Can you work these out from the model? Positions are in its coordinate system, mm. A direction names the side the tool comes from. Give positions to 0.01 mm unless a question says otherwise; leave off trailing zeros. Write each loop counter-clockwise with the first axis right and the second up, starting at its lowest first coordinate (ties: lowest second). Pieces come first, ordered by that corner, then holes.
Autodesk Inventor part; units mm, degrees
ref_plane "YZ Plane" through (0, 0, 0) normal (1, 0, 0) x (0, 1, 0)
ref_plane "XZ Plane" through (0, 0, 0) normal (0, 1, 0) x (-1, 0, 0)
ref_plane "XY Plane" through (0, 0, 0) normal (0, 0, 1) x (1, 0, 0)
sketch "Sketch1" plane through (0, 0, 0) normal (0, 1, 0) x (-1, 0, 0)
  circle A0 centre (0, 0) radius 4.25
  dimension "d0" = 8.5
extrude "Extrusion1" add sketch "Sketch1" along normal blind 2.5
sketch "Sketch2" plane through (0, 0, 0) normal (0, -1, 0) x (1, 0, 0)
  circle A0 centre (0, 0) radius 5.5
  dimension "d3" = 11
extrude "Extrusion2" add sketch "Sketch2" along normal blind 2.7
fillet "Fillet1" radius 1 1 edges at (4.25, 2.5, 0)
chamfer "Chamfer1" distance 2 angle 45 1 edges at (-5.5, -2.7, 0)
properties part number "button_round_3DPrint"
1) Suppose I cut it at B-B on z = 0. Write out the boundary of the cut face in (x, y).
Values follow:
outline: (-5.5, -0.7) - (-3.5, -2.7) - (3.5, -2.7) - (5.5, -0.7) - (5.5, 0) - (4.25, 0) - (4.25, 1.5) arc R1 ccw to (3.25, 2.5) - (-3.25, 2.5) arc R1 ccw to (-4.25, 1.5) - (-4.25, 0) - (-5.5, 0) - close
2) Suppose I cut it at C-C on y = -1.3. Write out the boundary of the cut face in (x, z).
Values follow:
outline: circle Ø9.8 at (0, 0)
3) For faces 1 (the face through (-2.285, 0.74, -3.584)), 2 (the face through (0, 2.5, 0)), which set-ups out of +Z, -Z, +X, -X, +Y, -Y let a thin tool reach every point of the face, with its end or its side?
Values follow:
face 1: +Y
face 2: +Z, -Z, +X, -X, +Y
4) Suppose I cut it at D-D on y = -2.35. Write out the boundary of the cut face in (x, z).
Values follow:
outline: circle Ø7.7 at (0, 0)
5) For pin 1 Ø2 at (x, z) = (4.5, 3) entering from +Y; pin 2 Ø1 at (x, z) = (4.5, 0.5) entering from +Y; pin 3 Ø1.5 at (y, z) = (2, -1.5) entering from -X; pin 4 Ø1.5 at (x, z) = (-1.5, 3) entering from +Y, each with a flat end and sliding along its axis, tell me the tip position at first contact or that it passes through.
Values follow:
pin 1: stops at y = 0
pin 2: stops at y = 2.13
pin 3: stops at x = -4.16
pin 4: stops at y = 2.5
6) Suppose I cut it at A-A on x = 0. Write out the boundary of the cut face in (y, z).
Values follow:
outline: (-2.7, -3.5) - (-0.7, -5.5) - (0, -5.5) - (0, -4.25) - (1.5, -4.25) arc R1 ccw to (2.5, -3.25) - (2.5, 3.25) arc R1 ccw to (1.5, 4.25) - (0, 4.25) - (0, 5.5) - (-0.7, 5.5) - (-2.7, 3.5) - close
7) Please list where these lines run through material, in increasing order: L1, parallel to Z at x = 2.75, y = -1.1; L2, parallel to Y at x = 4.5, z = -0.5; L3, parallel to X at y = -1.95, z = 3.25.
Values follow:
L1: z = -4.3 to 4.3
L2: y = -1.67 to 0
L3: x = -2.74 to 2.74
